Verification items for the finished model (mm, model axes). A direction names the side the tool comes from. Coordinates: 2 decimals unless noted, no trailing zeros. Write each loop counter-clockwise with the first axis right and the second up, starting at its lowest first coordinate (ties: lowest second). Pieces come first, ordered by that corner, then holes. Notation, with made-up numbers: (65.5, 16.5) - (99.5, 16.5) arc R10 cw to (99.5, 27.5) - close; hole circle Ø7 at (76.25, 23.25). An arc over 180 degrees is marked (long way). Use one line per item in the form item = value. Start each with the question number.
(1) Gauge pin test, flat ends, axial feed: pin 1 Ø5.5 at (x, z) = (4.5, -4) entering from +Y; pin 2 Ø1.8 at (y, z) = (55.5, -4) entering from +X; pin 3 Ø3 at (x, y) = (3, 57.5) entering from -Z. Record the tip position at first contact, or that the pin passes through.
(2) Sectioned sample at C-C (x = 8.25). Record the cut outline in (y, z), and give its area (3 significant figures).
(3) Sectioned sample at B-B (y = 21). Record the cut outline in (x, z), and give its area (3 significant figures).
(4) Sectioned sample at A-A (z = -3). Record the cut outline in (x, y), and give its area (3 significant figures).
(5) Tool access check on faces 4 (the flat face through (5, 55, 3)), 5 (the flat face through (4, 30, 8)), 6 (the flat face through (4.1, 18, 0)). Record the directions out of +Z, -Z, +X, -X, +Y, -Y that give a thin tool (end or side, any length) a straight path to the whole face; none if there is none.
(6) Material ranges on line 1 (X direction, y = 20, z = 1); line 2 (Y direction, x = -1.25, z = -4.25); line 3 (Y direction, x = -3.5, z = -4.5), recorded low to high. Write a range as [from, to].
(7) Mould release check, pull along X, two halves, no side actions. Record for faces 1 (the flat face through (-10, 30, 0)), 2 (the cylindrical face through (0.1, 3.9, 0.1)), 3 (the cylindrical face through (-3, 55, 2)): released by +X, released by -X, zero draft, split by the parting line, or undercut.
(8) Sectioned sample at D-D (z = 4.5). Record the cut outline in (x, y).
from build123d import *

# Parameters (mm, degrees)
SKETCH1_W           = 20
SKETCH1_H           = 60
BOSS_EXTRUDE1_DEPTH = 8
CUT_EXTRUDE1_DEPTH  = 10


with BuildPart() as part:
    # Sketch1 → Boss-Extrude1 (new body, symmetric)
    with BuildSketch(Plane.XY):
        with Locations((0, 30)):
            Rectangle(SKETCH1_W, SKETCH1_H)
        with BuildLine():
            Line((4.1, 28), (4.1, 8))
            ThreePointArc((4.1, 8), (0, 3.9), (-4.1, 8))
            Line((-4.1, 8), (-4.1, 28))
            ThreePointArc((-4.1, 28), (0, 32.1), (4.1, 28))
        make_face(mode=Mode.SUBTRACT)
    extrude(amount=BOSS_EXTRUDE1_DEPTH, both=True)

    # Sketch2 → Cut-Extrude1 (cut)
    with BuildSketch(Plane(origin=(0, 60, 0), x_dir=(1, 0, 0), z_dir=(0, 1, 0))):
        with BuildLine():
            Line((10, -3), (0, -3))
            ThreePointArc((0, -3), (-3.535533906, -1.535533906), (-5, 2))
            Line((-5, 2), (-5, 8))
            Line((-5, 8), (10, 8))
            Line((10, 8), (10, -3))
        make_face()
    extrude(amount=-CUT_EXTRUDE1_DEPTH, mode=Mode.SUBTRACT)


solid = part.part
Answers below:
q1.pin_1 = 50
q1.pin_2 = -5
q1.pin_3 = 3
q2.outline = (0, -8) - (50, -8) - (50, 3) - (60, 3) - (60, 8) - (0, 8) - close
q2.area = 850 mm2
q3.outline = (-10, -8) - (-4.1, -8) - (-4.1, 8) - (-10, 8) - close; (4.1, -8) - (10, -8) - (10, 8) - (4.1, 8) - close
q3.area = 189 mm2
q4.outline = (-10, 0) - (10, 0) - (10, 50) - (-5, 50) - (-5, 60) - (-10, 60) - close; hole (-4.1, 8) arc R4.1 ccw to (4.1, 8) - (4.1, 28) arc R4.1 ccw to (-4.1, 28) - close
q4.area = 833 mm2
q5.face_4 = -Z, +X, +Y
q5.face_5 = +Z, +X, -X, +Y, -Y
q5.face_6 = +Z, -Z
q6.line_1 = [-10, -4.1], [4.1, 10]
q6.line_2 = [0, 4.1], [31.9, 50]
q6.line_3 = [0, 5.86], [30.14, 50]
q7.face_1 = released by -X
q7.face_2 = undercut
q7.face_3 = released by +X
q8.outline = (-10, 0) - (10, 0) - (10, 60) - (-10, 60) - close; hole (-4.1, 8) arc R4.1 ccw to (4.1, 8) - (4.1, 28) arc R4.1 ccw to (-4.1, 28) - close
